from build123d import *
from OCP.BRepFilletAPI import BRepFilletAPI_MakeChamfer

# Parameters (mm, degrees)
SKETCH1_W           = 65
SKETCH1_H           = 100
BOSS_EXTRUDE1_DEPTH = 2
SKETCH2_W           = 65
SKETCH2_H           = 100
SKETCH2_W_2         = 57
SKETCH2_H_2         = 92
BOSS_EXTRUDE2_DEPTH = 3
FILLET1_R           = 5
BOSS_EXTRUDE3_DEPTH = 10
SKETCH6_R           = 18
BOSS_EXTRUDE4_DEPTH = 5
CHAMFER1_SIZE       = 10
SKETCH7_R           = 13
CUT_EXTRUDE1_DEPTH  = 80.726093596
BOSS_EXTRUDE6_DEPTH = 2
BOSS_EXTRUDE7_DEPTH = 7
CHAMFER2_SIZE       = 1.3
CHAMFER2_SIZE2      = 4.000988598


with BuildPart() as part:
    # Sketch1 → Boss-Extrude1 (new body)
    with BuildSketch(Plane(origin=(0, 0, 0), x_dir=(1, 0, 0), z_dir=(0, 1, 0))):
        with Locations((0, -20)):
            Rectangle(SKETCH1_W, SKETCH1_H)
    extrude(amount=BOSS_EXTRUDE1_DEPTH)

    # Sketch2 → Boss-Extrude2 (add)
    with BuildSketch(Plane(origin=(0, 2, 0), x_dir=(1, 0, 0), z_dir=(0, 1, 0))):
        with Locations((0, -20)):
            Rectangle(SKETCH2_W, SKETCH2_H)
        with Locations((0, -20)):
            Rectangle(SKETCH2_W_2, SKETCH2_H_2, mode=Mode.SUBTRACT)
    extrude(amount=BOSS_EXTRUDE2_DEPTH)

    # Fillet1
    fillet1_edges = [part.edges().sort_by_distance(p)[0] for p in [
        (-28.5, 3.5, 66),
        (28.5, 3.5, 66),
        (28.5, 3.5, -26),
        (-28.5, 3.5, -26),
        (-32.5, 2.5, -30),
        (32.5, 2.5, -30),
        (32.5, 2.5, 70),
        (-32.5, 2.5, 70),
    ]]
    fillet(fillet1_edges, radius=FILLET1_R)

    # Sketch4 → Boss-Extrude3 (add)
    with BuildSketch(Plane(origin=(0, 5, 0), x_dir=(1, 0, 0), z_dir=(0, 1, 0))):
        with BuildLine():
            Line((-32.5, 25), (-32.5, -65))
            ThreePointArc((-32.5, -65), (-31.035533906, -68.535533906), (-27.5, -70))
            Line((-27.5, -70), (27.5, -70))
            ThreePointArc((27.5, -70), (31.035533906, -68.535533906), (32.5, -65))
            Line((32.5, -65), (32.5, 25))
            ThreePointArc((32.5, 25), (31.035533906, 28.535533906), (27.5, 30))
            Line((27.5, 30), (-27.5, 30))
            ThreePointArc((-27.5, 30), (-31.035533906, 28.535533906), (-32.5, 25))
        make_face()
        with BuildLine():
            Line((-30.5, 25), (-30.5, -65))
            ThreePointArc((-30.5, -65), (-29.621320344, -67.121320344), (-27.5, -68))
            Line((-27.5, -68), (27.5, -68))
            ThreePointArc((27.5, -68), (29.621320344, -67.121320344), (30.5, -65))
            Line((30.5, -65), (30.5, 25))
            ThreePointArc((30.5, 25), (29.621320344, 27.121320344), (27.5, 28))
            Line((27.5, 28), (-27.5, 28))
            ThreePointArc((-27.5, 28), (-29.621320344, 27.121320344), (-30.5, 25))
        make_face(mode=Mode.SUBTRACT)
    extrude(amount=BOSS_EXTRUDE3_DEPTH)

    # Sketch6 → Boss-Extrude4 (add)
    with BuildSketch(Plane(origin=(0, -5, 0), x_dir=(-1, 0, 0), z_dir=(0, -1, 0))):
        with Locations(Location((0, 0, 0), (0, 0, 90))):
            Circle(SKETCH6_R)
    extrude(amount=-BOSS_EXTRUDE4_DEPTH)

    # Chamfer1
    # the kernel refuses this chamfer: 10 mm, written as the material it adds along each edge
    with BuildSketch(Plane(origin=(0, 0, 0), x_dir=(0, 0, -1), z_dir=(-1, 0, 0))) as chamfer1_piece_1_section:
        Polygon((18 + CHAMFER1_SIZE, 0), (18, CHAMFER1_SIZE), (18, 0), align=None)
    chamfer1_piece_1 = revolve(axis=Axis((0, 0, 0), (0, -1, 0)), mode=Mode.PRIVATE)
    chamfer1_piece_1 = split(chamfer1_piece_1, bisect_by=Plane(origin=(0, -5, 25.515578953), z_dir=(0, 1, 0)), keep=Keep.TOP, mode=Mode.PRIVATE)
    add(chamfer1_piece_1)

    # Sketch7 → Cut-Extrude1 (cut, through all)
    with BuildSketch(Plane.XZ.offset(5)):
        with Locations(Location((0, 0, 0), (0, 0, 270))):
            Circle(SKETCH7_R)
    extrude(amount=-CUT_EXTRUDE1_DEPTH, mode=Mode.SUBTRACT)

    # Sketch8 → Boss-Extrude6 (add)
    with BuildSketch(Plane(origin=(0, -5, 0), x_dir=(-1, 0, 0), z_dir=(0, -1, 0))):
        with BuildLine():
            ThreePointArc((-9.53952181, 6.422423502), (-4.636164201, 10.524066776), (1.699808228, 11.373682429))
            Line((1.699808228, 11.373682429), (1.921522345, 12.857206224))
            ThreePointArc((1.921522345, 12.857206224), (-5.240881271, 11.896771138), (-10.783807263, 7.260130916))
            Line((-10.783807263, 7.260130916), (-9.53952181, 6.422423502))
        make_face()
        with BuildLine():
            Line((1.921522345, 12.857206224), (1.699808228, 11.373682429))
            ThreePointArc((1.699808228, 11.373682429), (4.307975824, 10.662614328), (6.678083991, 9.362328461))
            Line((6.678083991, 9.362328461), (7.549138424, 10.583501739))
            ThreePointArc((7.549138424, 10.583501739), (4.869885714, 12.053390109), (1.921522345, 12.857206224))
        make_face()
        with BuildLine():
            Line((12.464656553, 3.692199481), (11.026426951, 3.266176464))
            ThreePointArc((11.026426951, 3.266176464), (11.380990948, 1.650165153), (11.5, 0))
            ThreePointArc((11.5, 0), (10.443646499, -4.814586982), (7.468652556, -8.744668604))
            Line((7.468652556, -8.744668604), (8.442824628, -9.885277553))
            ThreePointArc((8.442824628, -9.885277553), (11.80586126, -5.442576588), (13, 0))
            ThreePointArc((13, 0), (12.865468029, 1.865404086), (12.464656553, 3.692199481))
        make_face()
        with BuildLine():
            ThreePointArc((7.468652556, -8.744668604), (6.263348903, -9.644711531), (4.950877613, -10.37973077))
            Line((4.950877613, -10.37973077), (5.596644259, -11.733608697))
            ThreePointArc((5.596644259, -11.733608697), (7.080307455, -10.902717383), (8.442824628, -9.885277553))
            Line((8.442824628, -9.885277553), (7.468652556, -8.744668604))
        make_face()
        with BuildLine():
            ThreePointArc((-8.917379083, 6.003569796), (-4.333805666, 9.837714595), (1.58895117, 10.631920531))
            Line((1.58895117, 10.631920531), (1.699808228, 11.373682429))
            ThreePointArc((1.699808228, 11.373682429), (-4.636164201, 10.524066776), (-9.53952181, 6.422423502))
            Line((-9.53952181, 6.422423502), (-8.917379083, 6.003569796))
        make_face()
        with BuildLine():
            Line((11.026426951, 3.266176464), (10.30731215, 3.053164956))
            ThreePointArc((10.30731215, 3.053164956), (10.638752408, 1.542545686), (10.75, 0))
            ThreePointArc((10.75, 0), (9.762539119, -4.500592179), (6.98156652, -8.17436413))
            Line((6.98156652, -8.17436413), (7.468652556, -8.744668604))
            ThreePointArc((7.468652556, -8.744668604), (10.443646499, -4.814586982), (11.5, 0))
            ThreePointArc((11.5, 0), (11.380990948, 1.650165153), (11.026426951, 3.266176464))
        make_face()
        with BuildLine():
            Line((-2.48051694, -12.761153385), (-2.194303447, -11.28871261))
            ThreePointArc((-2.194303447, -11.28871261), (-7.98857126, -8.272407704), (-11.205255745, -2.586937125))
            Line((-11.205255745, -2.586937125), (-12.666810842, -2.924363706))
            ThreePointArc((-12.666810842, -2.924363706), (-9.030558816, -9.351417404), (-2.48051694, -12.761153385))
        make_face()
        with BuildLine():
            Line((-2.194303447, -11.28871261), (-2.0511967, -10.552492222))
            ThreePointArc((-2.0511967, -10.552492222), (-7.467577482, -7.732902854), (-10.474478196, -2.418223834))
            Line((-10.474478196, -2.418223834), (-11.205255745, -2.586937125))
            ThreePointArc((-11.205255745, -2.586937125), (-7.98857126, -8.272407704), (-2.194303447, -11.28871261))
        make_face()
        with BuildLine():
            ThreePointArc((-11.205255745, -2.586937125), (-11.451756667, -1.052268615), (-11.489054548, 0.501622955))
            Line((-11.489054548, 0.501622955), (-12.987626881, 0.567052036))
            ThreePointArc((-12.987626881, 0.567052036), (-12.945464058, -1.189521043), (-12.666810842, -2.924363706))
            Line((-12.666810842, -2.924363706), (-11.205255745, -2.586937125))
        make_face()
    extrude(amount=-BOSS_EXTRUDE6_DEPTH)

    # Sketch8<5> → Boss-Extrude7 (add)
    with BuildSketch(Plane(origin=(0, -5, 0), x_dir=(-1, 0, 0), z_dir=(0, -1, 0))):
        with BuildLine():
            Line((1.921522345, 12.857206224), (1.699808228, 11.373682429))
            ThreePointArc((1.699808228, 11.373682429), (4.307975824, 10.662614328), (6.678083991, 9.362328461))
            Line((6.678083991, 9.362328461), (7.549138424, 10.583501739))
            ThreePointArc((7.549138424, 10.583501739), (4.869885714, 12.053390109), (1.921522345, 12.857206224))
        make_face()
        with BuildLine():
            ThreePointArc((7.468652556, -8.744668604), (6.263348903, -9.644711531), (4.950877613, -10.37973077))
            Line((4.950877613, -10.37973077), (5.596644259, -11.733608697))
            ThreePointArc((5.596644259, -11.733608697), (7.080307455, -10.902717383), (8.442824628, -9.885277553))
            Line((8.442824628, -9.885277553), (7.468652556, -8.744668604))
        make_face()
        with BuildLine():
            ThreePointArc((-11.205255745, -2.586937125), (-11.451756667, -1.052268615), (-11.489054548, 0.501622955))
            Line((-11.489054548, 0.501622955), (-12.987626881, 0.567052036))
            ThreePointArc((-12.987626881, 0.567052036), (-12.945464058, -1.189521043), (-12.666810842, -2.924363706))
            Line((-12.666810842, -2.924363706), (-11.205255745, -2.586937125))
        make_face()
    extrude(amount=-BOSS_EXTRUDE7_DEPTH)

    # Chamfer2: one chamfer whose edges measure the first distance from different faces: ONE call of the kernel's chamfer builder (chamfer() names one face for all edges)
    chamfer2_edges_1 = [part.edges().sort_by_distance(p)[0] for p in [
        (9.850593173, -3, -6.631850356),
    ]]
    chamfer2_side_1 = [part.faces().sort_by_distance(p)[0] for p in [
        (9.850593173, -4, -6.631850356),
    ]]
    chamfer2_edges_2 = [part.edges().sort_by_distance(p)[0] for p in [
        (-11.385984352, -3, -3.372682218),
    ]]
    chamfer2_side_2 = [part.faces().sort_by_distance(p)[0] for p in [
        (-11.385984352, -4, -3.372682218),
    ]]
    chamfer2_edges_3 = [part.edges().sort_by_distance(p)[0] for p in [
        (2.26585682, -3, 11.656822803),
    ]]
    chamfer2_side_3 = [part.faces().sort_by_distance(p)[0] for p in [
        (2.26585682, -4, 11.656822803),
    ]]
    chamfer2 = BRepFilletAPI_MakeChamfer(part.part.solid().wrapped)
    for e in chamfer2_edges_1:
        chamfer2.Add(CHAMFER2_SIZE, CHAMFER2_SIZE2, e.wrapped, chamfer2_side_1[0].wrapped)  # the first distance lies on this face
    for e in chamfer2_edges_2:
        chamfer2.Add(CHAMFER2_SIZE, CHAMFER2_SIZE2, e.wrapped, chamfer2_side_2[0].wrapped)  # the first distance lies on this face
    for e in chamfer2_edges_3:
        chamfer2.Add(CHAMFER2_SIZE, CHAMFER2_SIZE2, e.wrapped, chamfer2_side_3[0].wrapped)  # the first distance lies on this face
    add(Compound.cast(chamfer2.Shape()), mode=Mode.REPLACE)


solid = part.part
The model under review builds one solid part; all positions refer to its coordinate system, in mm. A direction names the side the tool comes from. Coordinates: 2 decimals unless noted, no trailing zeros. Loops run counter-clockwise (first coordinate to the right, second up) from the corner with the lowest first, then second, coordinate; pieces in that order, holes last.
(1) Draft analysis for pull direction X (two halves, no side actions). For faces 4 (the flat face through (31, 15, 5)), 5 (the flat face through (-32.5, 7, 19)), 6 (the flat face through (3, -3, -11)), state which applies: +X half, -X half, draft (parallel to the pull), parting line (faces both ways), or undercut.
Determined:
face 4: draft
face 5: -X half
face 6: undercut
(2) Consider section B-B, the plane x = 0. Give the boundary of the cut face in (y, z), plus the area to 4 significant figures.
Determined:
outline: (-5, -23) - (0, -28) - (0, -30) - (15, -30) - (15, -28) - (5, -28) - (5, -26) - (2, -26) - (2, -13) - (-3, -13) - (-3, -10.75) - (-5, -10.75) - close; (-5, 13) - (2, 13) - (2, 66) - (5, 66) - (5, 68) - (15, 68) - (15, 70) - (0, 70) - (0, 28) - (-5, 23) - close
area: 341.5 mm2
(3) Insertion check: P1, Ø3.5, axis at x = 9.5, z = 7, coming from the +Y side; P2, Ø2, axis at x = 4, z = -10.5, coming from the +Y side; P3, Ø8, axis at x = -14.5, z = 18, coming from the -Y side. Each pin has a flat end and moves straight along its axis. Give the tip position at first contact, or say it passes through.
Determined:
P1: stops at y = 2
P2: stops at y = -3
P3: stops at y = -5
(4) Wall thickness on L1, parallel to Z at x = -17, y = 3.5; L2, parallel to X at y = 11, z = 17; L3, parallel to Z at x = 10.5, y = 9.75: over which ranges is each line inside the solid? List them lowest first.
Determined:
L1: z = -30 to -26, 66 to 70
L2: x = -32.5 to -30.5, 30.5 to 32.5
L3: z = -30 to -28, 68 to 70
(5) Tool access review of faces 1 (the cylindrical face through (7.4, -4, 7.8)), 2 (the flat face through (0, 7, -30)), 3 (the flat face through (-11, -3, 5)): name each direction out of +Z, -Z, +X, -X, +Y, -Y from which nothing blocks a thin tool from reaching the whole face with its end or side.
Determined:
face 1: +Y, -Y
face 2: -Z, +X, -X, +Y, -Y
face 3: +Y
(6) Consider section A-A, the plane y = 11. Give the boundary of the cut face in (x, z).
Determined:
outline: (-32.5, -25) arc R5 ccw to (-27.5, -30) - (27.5, -30) arc R5 ccw to (32.5, -25) - (32.5, 65) arc R5 ccw to (27.5, 70) - (-27.5, 70) arc R5 ccw to (-32.5, 65) - close; hole (-30.5, -25) arc R3 ccw to (-27.5, -28) - (27.5, -28) arc R3 ccw to (30.5, -25) - (30.5, 65) arc R3 ccw to (27.5, 68) - (-27.5, 68) arc R3 ccw to (-30.5, 65) - close
(7) Consider section C-C, the plane z = 47. Give the boundary of the cut face in (x, y), plus the area to 3 significant figures.
Determined:
outline: (-32.5, 0) - (32.5, 0) - (32.5, 15) - (30.5, 15) - (30.5, 5) - (28.5, 5) - (28.5, 2) - (-28.5, 2) - (-28.5, 5) - (-30.5, 5) - (-30.5, 15) - (-32.5, 15) - close
area: 194 mm2
